Check sheet for the modelled part. Datum: model origin and axes. Units: mm. A direction names the side the tool comes from. Round coordinates to 2 decimals unless told otherwise and drop trailing zeros. Write each loop counter-clockwise with the first axis right and the second up, starting at its lowest first coordinate (ties: lowest second). Pieces come first, ordered by that corner, then holes. Notation, with made-up numbers: (77, 36) -> (132, 36) arc R22 ccw to (132, 63) -> close; hole circle Ø4 at (19, 26). An arc over 180 degrees is marked (long way). One line per item, written item: value.
from build123d import *

# Parameters (mm, degrees)
SKETCH1_W               = 50
SKETCH1_H               = 10
BOSS_EXTRUDE1_DEPTH     = 10
SKETCH2_W               = 30
SKETCH2_H               = 10
CUT_EXTRUDE1_DEPTH      = 6
FILLET3_R               = 5
CUT_EXTRUDE2_DEPTH      = 42.533119315
CUT_EXTRUDE2_DEPTH_BACK = 42.533119315
SKETCH3_R               = 1.25
FILLET4_R               = 5
SKETCH4_W               = 10
SKETCH4_H               = 37.18
BOSS_EXTRUDE2_DEPTH     = 15
FILLET7_R               = 2.5
SKETCH5_W               = 10
SKETCH5_H               = 27.18
CUT_EXTRUDE3_DEPTH      = 10
FILLET8_R               = 2.5
CUT_EXTRUDE4_DEPTH      = 48.807451302
CUT_EXTRUDE4_DEPTH_BACK = 48.807451302
SKETCH6_R               = 1.25
FILLET9_R               = 3.5
FILLET10_R              = 5
FILLET11_R              = 3


with BuildPart() as part:
    # Sketch1 → Boss-Extrude1 (new body)
    with BuildSketch(Plane(origin=(0, 0, 0), x_dir=(1, 0, 0), z_dir=(0, 1, 0))):
        Rectangle(SKETCH1_W, SKETCH1_H)
    extrude(amount=BOSS_EXTRUDE1_DEPTH)

    # Sketch2 → Cut-Extrude1 (cut)
    with BuildSketch(Plane.XZ):
        Rectangle(SKETCH2_W, SKETCH2_H)
    extrude(amount=-CUT_EXTRUDE1_DEPTH, mode=Mode.SUBTRACT)

    # Fillet3
    fillet3_edges = [part.edges().sort_by_distance(p)[0] for p in [
        (-20, 0, -5),
        (20, 0, -5),
        (20, 0, 5),
        (-20, 0, 5),
    ]]
    fillet(fillet3_edges, radius=FILLET3_R - 0.0001)  # a hair under: the kernel refuses the full size

    # Sketch3 → Cut-Extrude2 (cut, two sides: drawn at the far end of the back side and taken through both)
    with BuildSketch(Plane(origin=(-15, 0, 0), x_dir=(0, 0, -1), z_dir=(1, 0, 0)).offset(-CUT_EXTRUDE2_DEPTH_BACK)):
        with Locations((0, 1.464466094)):
            Circle(SKETCH3_R)
    extrude(amount=CUT_EXTRUDE2_DEPTH + CUT_EXTRUDE2_DEPTH_BACK, mode=Mode.SUBTRACT)

    # Fillet4
    fillet4_edges = [part.edges().sort_by_distance(p)[0] for p in [
        (25, 10, 0),
        (-25, 10, 0),
    ]]
    fillet(fillet4_edges, radius=FILLET4_R)

    # Sketch4 → Boss-Extrude2 (add)
    with BuildSketch(Plane(origin=(0, 10, 0), x_dir=(1, 0, 0), z_dir=(0, 1, 0))):
        Rectangle(SKETCH4_W, SKETCH4_H)
    extrude(amount=BOSS_EXTRUDE2_DEPTH)

    # Fillet7
    fillet7_edges = [part.edges().sort_by_distance(p)[0] for p in [
        (0, 10, 5),
        (0, 10, -5),
    ]]
    fillet(fillet7_edges, radius=FILLET7_R)

    # Sketch5 → Cut-Extrude3 (cut)
    with BuildSketch(Plane(origin=(0, 25, 0), x_dir=(1, 0, 0), z_dir=(0, 1, 0))):
        Rectangle(SKETCH5_W, SKETCH5_H)
    extrude(amount=-CUT_EXTRUDE3_DEPTH, mode=Mode.SUBTRACT)

    # Fillet8
    fillet8_edges = [part.edges().sort_by_distance(p)[0] for p in [
        (5, 10, 0),
        (-5, 10, 0),
    ]]
    fillet(fillet8_edges, radius=FILLET8_R)

    # Sketch6 → Cut-Extrude4 (cut, two sides: drawn at the far end of the back side and taken through both)
    with BuildSketch(Plane(origin=(0, 0, 13.59), x_dir=(-1, 0, 0), z_dir=(0, 0, -1)).offset(-CUT_EXTRUDE4_DEPTH_BACK)):
        with Locations((0, 23.464881358)):
            Circle(SKETCH6_R)
    extrude(amount=CUT_EXTRUDE4_DEPTH + CUT_EXTRUDE4_DEPTH_BACK, mode=Mode.SUBTRACT)

    # Fillet9
    fillet9_edges = [part.edges().sort_by_distance(p)[0] for p in [
        (-5, 25, 16.09),
        (5, 25, -16.09),
        (-5, 25, -16.09),
        (5, 25, 16.09),
    ]]
    fillet(fillet9_edges, radius=FILLET9_R)

    # Fillet10
    fillet10_edges = [part.edges().sort_by_distance(p)[0] for p in [
        (0, 10, 18.59),
        (0, 10, -18.59),
    ]]
    fillet(fillet10_edges, radius=FILLET10_R)

    # Fillet11
    fillet11_edges = [part.edges().sort_by_distance(p)[0] for p in [
        (0, 15, 13.59),
        (0, 15, -13.59),
    ]]
    fillet(fillet11_edges, radius=FILLET11_R)


solid = part.part
Item 1: Sectioned sample at B-B (y = 4.25). Enter the section's corners in (x, z).
Result set:
outline: (-25, -4.94) -> (-15, -4.94) -> (-15, 4.94) -> (-25, 4.94) -> close; (15, -4.94) -> (25, -4.94) -> (25, 4.94) -> (15, 4.94) -> close
Item 2: Material ranges on line 1 along Y through (x, z) = (-18.5, 0); line 2 along X through (y, z) = (11.5, -15); line 3 along Y through (x, z) = (-3, -1.5), recorded low to high.
Result set:
line 1: 0 to 0.21, 2.71 to 10
line 2: -5 to 5
line 3: 6 to 15
Item 3: Release check for a two-part mould opening along X. For faces 1 (the cylindrical face through (5.713, 10.752, -0.07)), 2 (the flat face through (0, 6, 0)), 3 (the cylindrical face through (0.271, 22.245, 16.125)), 4 (the cylindrical face through (20, 2, -4)) record: pulls with the +X half, pulls with the -X half, needs draft (parallel to the pull), parting line crosses it, or undercut.
Result set:
face 1: pulls with the +X half
face 2: undercut
face 3: undercut
face 4: needs draft
Item 4: Depth check by flat-ended pin: pin 1 (3 mm diameter, centred on x = 16.5, z = 0.5, fed in from +Y); pin 2 (8 mm diameter, centred on x = 0.5, z = 3, fed in from +Y); pin 3 (2 mm diameter, centred on x = -10.5, z = -5, fed in from -Y). Enter the tip coordinate at first touch or a pass-through.
Result set:
pin 1: y = 10
pin 2: y = 15
pin 3: y = 6
Item 5: Sectioned sample at A-A (x = 0). Enter the section's corners in (y, z).
Result set:
outline: (6, -5) -> (7.5, -5) arc R2.5 cw to (10, -7.5) -> (10, -13.59) arc R5 ccw to (15, -18.59) -> (22.21, -18.59) -> (22.21, -13.59) -> (18, -13.59) arc R3 cw to (15, -10.59) -> (15, 10.59) arc R3 cw to (18, 13.59) -> (22.21, 13.59) -> (22.21, 18.59) -> (15, 18.59) arc R5 ccw to (10, 13.59) -> (10, 7.5) arc R2.5 cw to (7.5, 5) -> (6, 5) -> close; (24.71, -18.59) -> (25, -18.59) -> (25, -13.59) -> (24.71, -13.59) -> close; (24.71, 13.59) -> (25, 13.59) -> (25, 18.59) -> (24.71, 18.59) -> close
Item 6: Sectioned sample at D-D (z = -10). Enter the section's corners in (x, y).
Result set:
outline: (-5, 10) -> (5, 10) -> (5, 15) -> (-5, 15) -> close
Item 7: Tool access check on faces 5 (the flat face through (0, 10, -11)), 6 (the flat face through (0, 21, 13.59)), 7 (the flat face through (-14, 10, 0)). Record the directions out of +Z, -Z, +X, -X, +Y, -Y that give a thin tool (end or side, any length) a straight path to the whole face; none if there is none.
Result set:
face 5: -Z, +X, -X, -Y
face 6: +X, -X, +Y
face 7: +Z, -Z, -X, +Y
